Can you work these out from the model? Positions are in its coordinate system, mm. Round coordinates to 2 decimals unless told otherwise and drop trailing zeros. Loops run counter-clockwise (first coordinate to the right, second up) from the corner with the lowest first, then second, coordinate; pieces in that order, holes last.
Autodesk Inventor part; units mm, degrees
ref_plane "YZ Plane" through (0, 0, 0) normal (1, 0, 0) x (0, 1, 0)
ref_plane "XZ Plane" through (0, 0, 0) normal (0, 1, 0) x (-1, 0, 0)
ref_plane "XY Plane" through (0, 0, 0) normal (0, 0, 1) x (1, 0, 0)
sketch "Esquisse1" plane through (0, 0, 0) normal (0, 0, 1) x (1, 0, 0)
  line L0 (-90, -44) -> (90, -44)
  line L1 (90, -44) -> (90, 44)
  line L2 (90, 44) -> (-90, 44)
  line L3 (-90, 44) -> (-90, -44)
  line L4 (-90, -44) -> (90, 44) construction
  line L5 (90, -44) -> (-90, 44) construction
  point P0 (0, 0)
  dimension "d0" = 180
  dimension "d1" = 88
extrude "Extrusion1" add sketch "Esquisse1" along normal mid plane 5
sketch "Esquisse2" plane through (0, 0, 2.5) normal (0, 0, 1) x (1, 0, 0)
  line L0 (-90, 44) -> (-90, -44)
  line L1 (90, -44) -> (-90, -44)
  point P0 (0, 0)
  point P1 (-45, -24)
  point P2 (-45, 9.85)
  point P3 (-11.15, 9.85)
  dimension "d4" = 33.85
  dimension "d5" = 45
  dimension "d6" = 33.85
  dimension "d7" = 20
hole "Perçage_moteur" at (-45, -24, 2.5) at (-45, 9.85, 2.5) at (-11.15, 9.85, 2.5) direction (0, 0, -1) diameter 4.2 end through all
sketch "Esquisse3" plane through (0, 0, 2.5) normal (0, 0, 1) x (1, 0, 0)
  line L0 (-60.0266, -12) -> (31.1582, -12) construction
  circle A0 centre (-45, -24) radius 2.1 construction
  circle A1 centre (-11.15, 9.85) radius 2.1 construction
  line L1 (-90, 44) -> (-90, -44)
  point P0 (0, 0)
  point P1 (8.85, -20)
  point P2 (8.85, -4)
  point P3 (48.85, -4)
  point P4 (48.85, -20)
  dimension "d15" = 40
  dimension "d16" = 16
  dimension "d17" = 12
  dimension "d18" = 8
  dimension "d19" = 20
  dimension "d38" = 98.85
hole "Perçage_laser" at (8.85, -20, 2.5) at (8.85, -4, 2.5) at (48.85, -4, 2.5) at (48.85, -20, 2.5) direction (0, 0, -1) diameter 3.2 depth 9.525 tip angle 118
sketch "Esquisse4" plane through (0, 0, 2.5) normal (0, 0, 1) x (1, 0, 0)
  line L0 (90, -44) -> (90, 44)
  line L1 (-90, 44) -> (90, 44)
  line L2 (90, -44) -> (-90, -44)
  line L3 (-90, 44) -> (-90, -44)
  point P0 (0, 0)
  point P1 (-80, -34)
  point P2 (-80, 34)
  point P3 (80, 34)
  point P4 (80, -34)
  dimension "d27" = 10
  dimension "d28" = 10
  dimension "d29" = 10
  dimension "d30" = 10
hole "Perçage_coins" at (-80, -34, 2.5) at (-80, 34, 2.5) at (80, 34, 2.5) at (80, -34, 2.5) direction (0, 0, -1) diameter 4.2 depth 9.525 tip angle 118
sketch "Esquisse5" plane through (0, 0, 2.5) normal (0, 0, 1) x (1, 0, 0)
  circle A0 centre (-45, 9.85) radius 2.1
  circle A1 centre (-11.15, 9.85) radius 2.1
  circle A2 centre (-45, -24) radius 2.1
  point P0 (0, 0)
  point P1 (-55, -24)
  point P2 (-55, 9.85)
  point P3 (-21.15, 9.85)
  dimension "d39" = 10
  dimension "d40" = 10
  dimension "d41" = 10
hole "Perçage4" at (-55, -24, 2.5) at (-55, 9.85, 2.5) at (-21.15, 9.85, 2.5) direction (0, 0, -1) diameter 4.2 depth 8 tip angle 118
equation "\"pi\" = 3.141593"
equation "\"nombredor\" = 1.61803"
properties part number "Plaque support" material "Aluminium 6061"
(1) Suppose I cut it at C-C (y = -34). Write out the boundary of the cut face in (x, z).
(2) Suppose I cut it at B-B (x = -80). Write out the boundary of the cut face in (y, z), then the cut area to 3 significant figures.
(3) Suppose I cut it at A-A (y = 9.85). Write out the boundary of the cut face in (x, z).
(4) For pin 1 (5.5 mm diameter, centred on x = -80, y = 34, fed in from -Z), with a flat end and sliding along its axis, tell me the tip position at first contact or that it passes through.
(5) Suppose I cut it at D-D (x = -21.15). Write out the boundary of the cut face in (y, z).
(6) If I drill on line 1 (X direction, y = 9.85, z = -0.35); line 2 (X direction, y = -24, z = 1.1); line 3 (X direction, y = -4, z = -0.7), over which ranges is the centre line in solid material (lowest first)?
(7) We'd pull the mould along Y, two halves only. Please class faces 1 (the flat face through (-1, 1, -2.5)), 2 (the cylindrical face through (-52.95, 10.31, -0.04)), 3 (the flat face through (1, 44, 0)): released by +Y, released by -Y, zero draft, split by the parting line, or undercut.
Check result:
1. outline: (-90, -2.5) - (-82.1, -2.5) - (-82.1, 2.5) - (-90, 2.5) - close; (-77.9, -2.5) - (77.9, -2.5) - (77.9, 2.5) - (-77.9, 2.5) - close; (82.1, -2.5) - (90, -2.5) - (90, 2.5) - (82.1, 2.5) - close
2. outline: (-44, -2.5) - (-36.1, -2.5) - (-36.1, 2.5) - (-44, 2.5) - close; (-31.9, -2.5) - (31.9, -2.5) - (31.9, 2.5) - (-31.9, 2.5) - close; (36.1, -2.5) - (44, -2.5) - (44, 2.5) - (36.1, 2.5) - close
2. area: 398 mm2
3. outline: (-90, -2.5) - (-57.1, -2.5) - (-57.1, 2.5) - (-90, 2.5) - close; (-52.9, -2.5) - (-47.1, -2.5) - (-47.1, 2.5) - (-52.9, 2.5) - close; (-42.9, -2.5) - (-23.25, -2.5) - (-23.25, 2.5) - (-42.9, 2.5) - close; (-19.05, -2.5) - (-13.25, -2.5) - (-13.25, 2.5) - (-19.05, 2.5) - close; (-9.05, -2.5) - (90, -2.5) - (90, 2.5) - (-9.05, 2.5) - close
4. pin 1: stops at z = -2.5
5. outline: (-44, -2.5) - (7.75, -2.5) - (7.75, 2.5) - (-44, 2.5) - close; (11.95, -2.5) - (44, -2.5) - (44, 2.5) - (11.95, 2.5) - close
6. line 1: x = -90 to -57.1, -52.9 to -47.1, -42.9 to -23.25, -19.05 to -13.25, -9.05 to 90
6. line 2: x = -90 to -57.1, -52.9 to -47.1, -42.9 to 90
6. line 3: x = -90 to 7.25, 10.45 to 47.25, 50.45 to 90
7. face 1: zero draft
7. face 2: undercut
7. face 3: released by +Y
